Job drawing, mm, ordinate dimensions from the low corner. One solid piece. Round coordinates to 2 decimals unless told otherwise and drop trailing zeros. Order: outer loops, then holes, each group sorted by start corner. A loop starts at its lowest first (then second) coordinate and runs counter-clockwise, first axis right, second up. Notation, with made-up numbers: (87.5, 62.5) -> (94.5, 62.5) arc R18 cw to (94.5, 93.5) -> close; hole circle Ø11 at (20, 3). An arc over 180 degrees is marked (long way). Return JSON: item names as keys, results as strings. Group by question number.
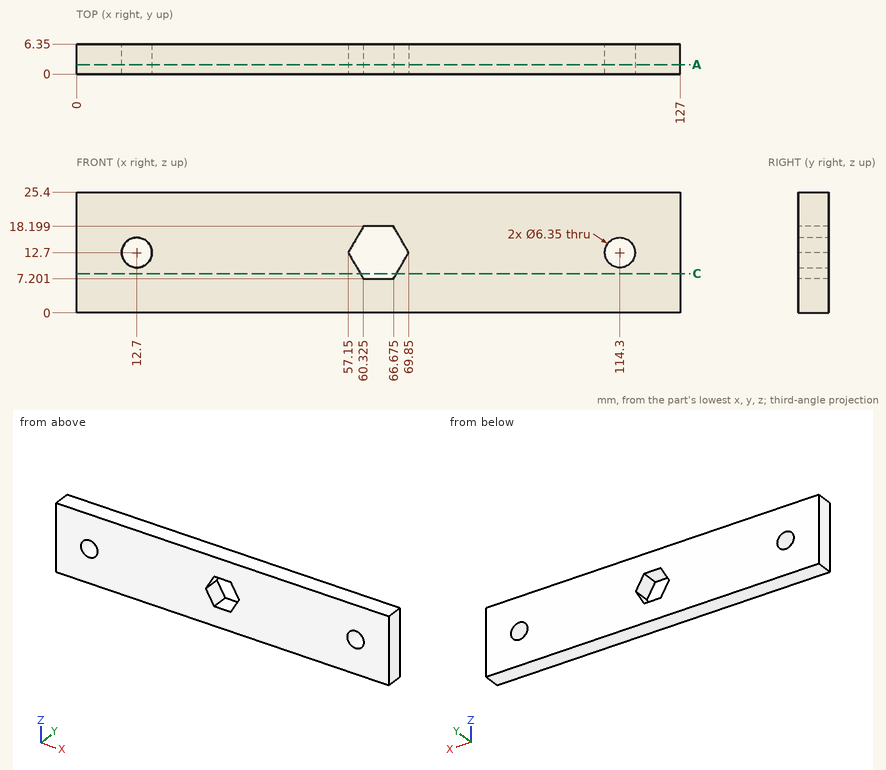
(1) Saw through at C-C, the plane z = 8.25. List the corners of the cut face in (x, y).
(2) Probe L1, parallel to Z at x = 114.3, y = 4.25 (1 decimal); L2, parallel to X at y = 1.5, z = 15; L3, parallel to Z at x = 12, y = 5.75. List the from-to ranges inside material, lowest first. Write a range as [from, to].
(3) Saw through at A-A, the plane y = 2. State how many separate pieces and enclosed holes the cut face has, and give its area (3 significant figures).
(4) Pin check, flat tip, straight feed: P1, Ø5, axis at x = 12.7, z = 12.7, coming from the -Y side. Stop position of the tip, or through.
Results are:
{
 "1": {"outline": "(0, 0) -> (59.72, 0) -> (59.72, 6.35) -> (0, 6.35) -> close; (67.28, 0) -> (127, 0) -> (127, 6.35) -> (67.28, 6.35) -> close"},
 "2": {"L1": "z = [0, 9.5], [15.9, 25.4]", "L2": "x = [0, 10.51], [14.89, 58.48], [68.52, 112.11], [116.49, 127]", "L3": "z = [0, 9.6], [15.8, 25.4]"},
 "3": {"separate pieces": "1", "enclosed holes": "3", "area": "3,060 mm^2"},
 "4": {"P1": "passes through"}
}
